```python
from build123d import *

# Parameters (mm, degrees)
SKETCH1_W                = 99
SKETCH1_H                = 56
SKETCH1_W_2              = 97
SKETCH1_H_2              = 54
SKETCH1_W_3              = 95
SKETCH1_H_3              = 52
BOSS_EXTRUDE1_DEPTH      = 2
SKETCH1_3_W              = 99
SKETCH1_3_H              = 56
SKETCH1_3_W_2            = 97
SKETCH1_3_H_2            = 54
BOSS_EXTRUDE2_DEPTH      = 10
SKETCH1_4_W              = 97
SKETCH1_4_H              = 54
SKETCH1_4_W_2            = 95
SKETCH1_4_H_2            = 52
BOSS_EXTRUDE3_DEPTH      = 8
F_3_0_3_DIAMETER_HOLE1_D = 3
CUT_EXTRUDE1_REACH       = 105.368
SKETCH7_W                = 20
SKETCH7_H                = 5
CUT_EXTRUDE2_REACH       = 77.407
SKETCH8_W                = 10
SKETCH8_H                = 5


with BuildPart() as part:
    # Sketch1 → Boss-Extrude1 (new body)
    with BuildSketch(Plane(origin=(0, 0, 0), x_dir=(1, 0, 0), z_dir=(0, 1, 0))):
        Rectangle(SKETCH1_W, SKETCH1_H)
        Rectangle(SKETCH1_W_2, SKETCH1_H_2, mode=Mode.SUBTRACT)
        Rectangle(SKETCH1_W_2, SKETCH1_H_2)
        Rectangle(SKETCH1_W_3, SKETCH1_H_3, mode=Mode.SUBTRACT)
        Polygon((47.5, 26), (-47.5, 26), (-47.5, -26), (-32.5, -26), (-32.5, 21), (2.5, 21), (2.5, -26), (47.5, -26), align=None)
    extrude(amount=BOSS_EXTRUDE1_DEPTH)

    # Sketch1<3> → Boss-Extrude2 (add)
    with BuildSketch(Plane(origin=(0, 0, 0), x_dir=(1, 0, 0), z_dir=(0, 1, 0))):
        Rectangle(SKETCH1_3_W, SKETCH1_3_H)
        Rectangle(SKETCH1_3_W_2, SKETCH1_3_H_2, mode=Mode.SUBTRACT)
    extrude(amount=-BOSS_EXTRUDE2_DEPTH)

    # Sketch1<4> → Boss-Extrude3 (add)
    with BuildSketch(Plane(origin=(0, 0, 0), x_dir=(1, 0, 0), z_dir=(0, 1, 0))):
        Rectangle(SKETCH1_4_W, SKETCH1_4_H)
        Rectangle(SKETCH1_4_W_2, SKETCH1_4_H_2, mode=Mode.SUBTRACT)
    extrude(amount=-BOSS_EXTRUDE3_DEPTH)

    # Ø3.0 (3) Diameter Hole1 (through all)
    with Locations(Plane(origin=(0, 0, 0), x_dir=(-1, 0, 0), z_dir=(0, -1, 0))):
        with Locations((-45, 21), (45, -21), (35, 21), (-5, -20)):
            Hole(F_3_0_3_DIAMETER_HOLE1_D / 2)

    # Cut-Extrude1: up to this face of the body (flat: up to its plane)
    cut_extrude1_end = Plane(part.part.faces().sort_by_distance((-47.5, -4, 0))[0])
    # Sketch7 → Cut-Extrude1 (cut, up to the picked face)
    with BuildSketch(Plane.ZY.offset(49.5), mode=Mode.PRIVATE) as cut_extrude1_sk1:
        with Locations((-2, -7.5)):
            Rectangle(SKETCH7_W, SKETCH7_H)
    cut_extrude1_tool1 = split(extrude(cut_extrude1_sk1.sketch, amount=-CUT_EXTRUDE1_REACH, mode=Mode.PRIVATE), bisect_by=cut_extrude1_end, keep=Keep.BOTH, mode=Mode.PRIVATE)
    add(cut_extrude1_tool1.solids().sort_by(Axis((-49.5, -7.5, -2), (1, 0, 0)))[0], mode=Mode.SUBTRACT)

    # Sketch8 → Cut-Extrude2 (cut, up to next)
    with BuildSketch(Plane(origin=(0, 0, -28), x_dir=(-1, 0, 0), z_dir=(0, 0, -1)), mode=Mode.PRIVATE) as cut_extrude2_sk1:
        with Locations((-24.5, -7.5)):
            Rectangle(SKETCH8_W, SKETCH8_H)
    cut_extrude2_tool1 = extrude(cut_extrude2_sk1.sketch, amount=-CUT_EXTRUDE2_REACH, mode=Mode.PRIVATE) & part.part
    add(cut_extrude2_tool1.solids().sort_by_distance((24.5, -7.5, -28))[0], mode=Mode.SUBTRACT)


solid = part.part
```
The model under review builds one solid part; all positions refer to its coordinate system, in mm. A direction names the side the tool comes from. Give positions to 0.01 mm unless a question says otherwise; leave off trailing zeros. Write each loop counter-clockwise with the first axis right and the second up, starting at its lowest first coordinate (ties: lowest second). Pieces come first, ordered by that corner, then holes.
(1) Tool access review of faces 1 (the flat face through (-49, -5, -2)), 2 (the flat face through (-32.5, 1, 3)), 3 (the flat face through (29.5, -7, -27)), 4 (the flat face through (39, -9, -27)): name each direction out of +Z, -Z, +X, -X, +Y, -Y from which nothing blocks a thin tool from reaching the whole face with its end or side.
(2) Consider section C-C, the plane x = -4.5. Give the boundary of the cut face in (y, z), and give its area (3 significant figures).
(3) Consider section D-D, the plane y = -1. Give the boundary of the cut face in (x, z), and give its area (3 significant figures).
(4) The part is to be moulded in two halves that separate along Z. For faces 5 (the flat face through (47.5, -4, 0)), 6 (the flat face through (-15, -9, -27)), 7 (the flat face through (25, -5, -27)), 8 (the flat face through (-1, -4, 28)), say which applies: released by +Z, released by -Z, zero draft, split by the parting line, or undercut.
(5) Consider section A-A, the plane y = -7. Give the boundary of the cut face in (x, z), and give its area (3 significant figures).
(6) To check wall thickness, follow L1, parallel to Z at x = 5, y = 0.6; L2, parallel to Z at x = -45, y = 1.1; L3, parallel to X at y = -1.25, z = 11. State the ranges of each line that lie inside material, in increasing order.
(7) Consider section B-B, the plane z = -15. Give the boundary of the cut face in (x, y).
(8) For P1, Ø3, axis at x = -0.5, z = -6.5, coming from the +Y side; P2, Ø3, axis at x = 21.5, y = -7.5, coming from the -Z side; P3, Ø4, axis at x = -45, z = 21, coming from the -Y side; P4, Ø1, axis at x = 23.5, z = -27, coming from the -Y side, all flat-tipped, find the tip position at first contact; note any pin that passes through.
Returned:
1. face 1: -X, -Y
1. face 2: +Y, -Y
1. face 3: -Z, -Y
1. face 4: -Y
2. outline: (-10, -28) - (2, -28) - (2, -21) - (0, -21) - (0, -26) - (-8, -26) - (-8, -27) - (-10, -27) - close; (-10, 27) - (-8, 27) - (-8, 26) - (2, 26) - (2, 28) - (-10, 28) - close
2. area: 54.0 mm2
3. outline: (-49.5, -28) - (49.5, -28) - (49.5, 28) - (-49.5, 28) - close; hole (-47.5, -26) - (47.5, -26) - (47.5, 26) - (-47.5, 26) - close
3. area: 604 mm2
4. face 5: undercut
4. face 6: undercut
4. face 7: zero draft
4. face 8: released by +Z
5. outline: (-49.5, -28) - (19.5, -28) - (19.5, -26) - (-47.5, -26) - (-47.5, -12) - (-49.5, -12) - close; (-49.5, 8) - (-47.5, 8) - (-47.5, 26) - (47.5, 26) - (47.5, -26) - (29.5, -26) - (29.5, -28) - (49.5, -28) - (49.5, 28) - (-49.5, 28) - close
5. area: 544 mm2
6. L1: z = -28 to 18.5, 21.5 to 28
6. L2: z = -28 to 19.5, 22.5 to 28
6. L3: x = -49.5 to -47.5, 47.5 to 49.5
7. outline: (-49.5, -10) - (-48.5, -10) - (-48.5, -8) - (-47.5, -8) - (-47.5, 0) - (-32.5, 0) - (-32.5, 2) - (-49.5, 2) - close; (2.5, 0) - (47.5, 0) - (47.5, -8) - (48.5, -8) - (48.5, -10) - (49.5, -10) - (49.5, 2) - (2.5, 2) - close
8. P1: passes through
8. P2: stops at z = 26
8. P3: stops at y = 0
8. P4: stops at y = -5
